Verification items for this drawing (mm, ordinates from the low corner). Give positions to 0.01 mm unless a question says otherwise; leave off trailing zeros. Write each loop counter-clockwise with the first axis right and the second up, starting at its lowest first coordinate (ties: lowest second). Pieces come first, ordered by that corner, then holes. Notation, with made-up numbers: (32, 73.25) -> (88, 73.25) arc R23 ccw to (88, 90.25) -> close; hole circle Ø9 at (19.5, 74.5). An arc over 180 degrees is marked (long way). One line per item, written item: value.
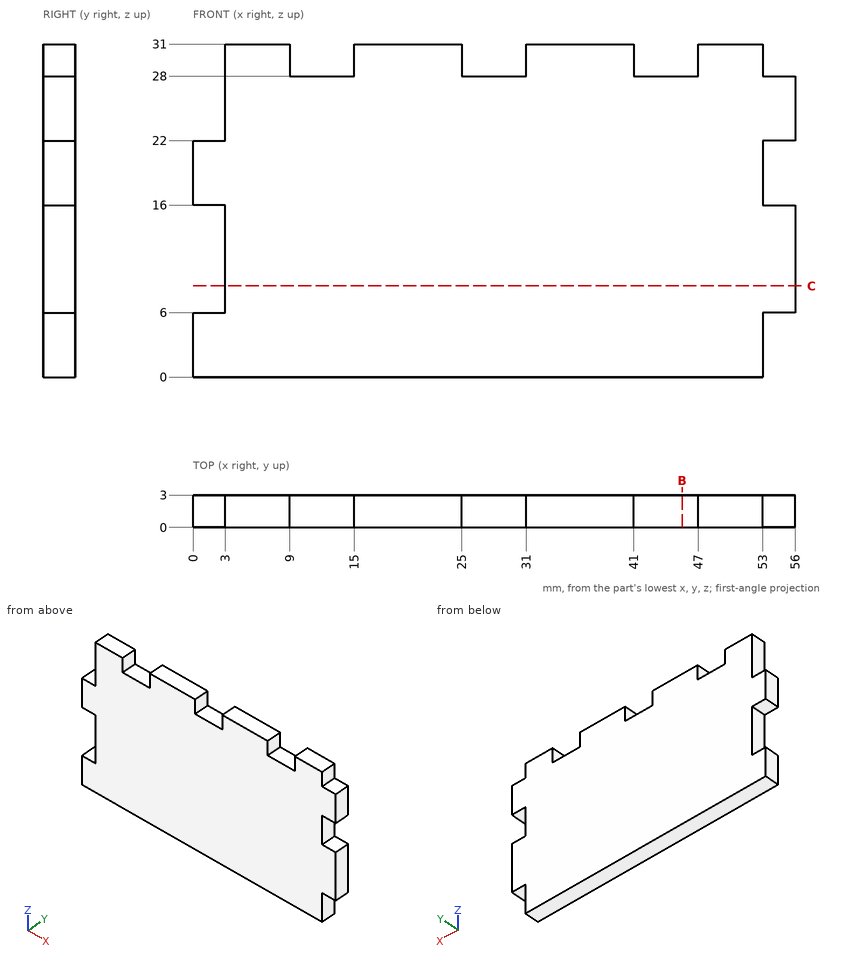
1) Sectioned sample at C-C on z = 8.5. Record the cut outline in (x, y).
Verdict:
outline: (3, 0) -> (56, 0) -> (56, 3) -> (3, 3) -> close
2) Scan lines: probe 1 along X at (y, z) = (0.7, 20); probe 2 along X at (y, z) = (1.65, 8); probe 3 along Z at (x, y) = (13, 0.65). Record each from-to range of solid material in increasing order.
Verdict:
probe 1: 0 to 53
probe 2: 3 to 56
probe 3: 0 to 28
3) Sectioned sample at B-B on x = 45.5. Record the cut outline in (y, z), plus the area to 3 significant figures.
Verdict:
outline: (0, 0) -> (3, 0) -> (3, 28) -> (0, 28) -> close
area: 84.0 mm^2
4) Depth check by flat-ended pin: pin 1 Ø1.5 at (x, y) = (44.5, 2) entering from +Z; pin 2 Ø1.5 at (y, z) = (1, 18) entering from +X; pin 3 Ø1.5 at (x, y) = (2, 1) entering from +Z. Enter the tip coordinate at first touch or a pass-through.
Verdict:
pin 1: z = 28
pin 2: x = 53
pin 3: z = 22
